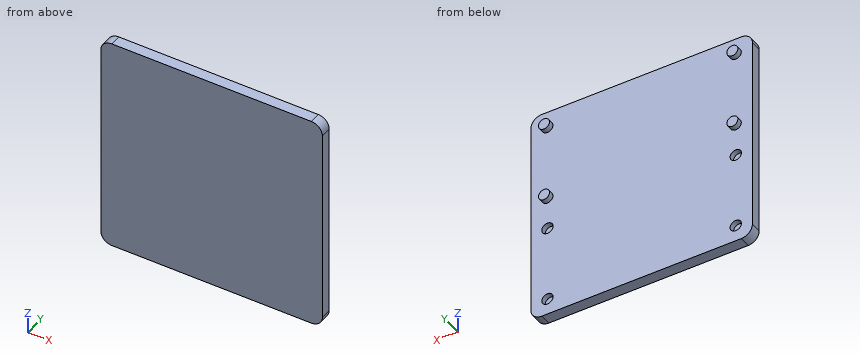
from build123d import *

# Parameters (mm, degrees)
SKETCH_1_W          = 200
SKETCH_1_H          = 200
EXTRUDE_1_DEPTH     = 10
SKETCH_2_R          = 5
EXTRUDE_2_DEPTH     = 5
FILLET_1_R          = 10
SKETCH_3_R          = 5.1
CUT_EXTRUDE_1_DEPTH = 5


with BuildPart() as part:
    # ｽｹｯﾁ1 → ﾎﾞｽ - 押し出し1 (new body)
    with BuildSketch(Plane(origin=(0, 0, 0), x_dir=(1, 0, 0), z_dir=(0, 1, 0))):
        Rectangle(SKETCH_1_W, SKETCH_1_H)
    extrude(amount=EXTRUDE_1_DEPTH)

    # ｽｹｯﾁ2 → ﾎﾞｽ - 押し出し2 (add)
    with BuildSketch(Plane(origin=(0, 10, 0), x_dir=(1, 0, 0), z_dir=(0, 1, 0))):
        with Locations(Location((-85, -15, 0), (0, 0, 90))):
            Circle(SKETCH_2_R)
        with Locations(Location((-85, -85, 0), (0, 0, 90))):
            Circle(SKETCH_2_R)
        with Locations(Location((85, -85, 0), (0, 0, 90))):
            Circle(SKETCH_2_R)
        with Locations(Location((85, -15, 0), (0, 0, 90))):
            Circle(SKETCH_2_R)
    extrude(amount=EXTRUDE_2_DEPTH)

    # ﾌｨﾚｯﾄ1
    fillet_1_edges = [part.edges().sort_by_distance(p)[0] for p in [
        (100, 5, 100),
        (-100, 5, 100),
        (-100, 5, -100),
        (100, 5, -100),
    ]]
    fillet(fillet_1_edges, radius=FILLET_1_R)

    # ｽｹｯﾁ3 → ｶｯﾄ - 押し出し1 (cut)
    with BuildSketch(Plane(origin=(0, 10, 0), x_dir=(1, 0, 0), z_dir=(0, 1, 0))):
        with Locations(Location((-85, 85, 0), (0, 0, 270))):
            Circle(SKETCH_3_R)
        with Locations(Location((85, 85, 0), (0, 0, 270))):
            Circle(SKETCH_3_R)
        with Locations(Location((-85, 15, 0), (0, 0, 270))):
            Circle(SKETCH_3_R)
        with Locations(Location((85, 15, 0), (0, 0, 270))):
            Circle(SKETCH_3_R)
    extrude(amount=-CUT_EXTRUDE_1_DEPTH, mode=Mode.SUBTRACT)


solid = part.part
The listing builds one solid part. Answer for the finished solid, in the listing's coordinates (mm). Coordinates: 2 decimals unless noted, no trailing zeros. Order: outer loops, then holes, each group sorted by start corner. A loop starts at its lowest first (then second) coordinate and runs counter-clockwise, first axis right, second up.
Q1. Consider line 1 (X direction, y = 8.6, z = -85); line 2 (Y direction, x = 46.5, z = -71); line 3 (Z direction, x = -86.5, y = 8.75). Determine where each line is inside the solid, lowest interval first.
Q2. A cutting plane is placed at A-A, the plane z = 85. Write down the section's boundary in (x, y).
Q3. A cutting plane is placed at D-D, the plane z = 53. Write down the section's boundary in (x, y).
Q4. Given P1, Ø2, axis at x = -35, z = -51.5, coming from the -Y side; P2, Ø11, axis at x = -85.5, z = -16.5, coming from the +Y side; P3, Ø5, axis at x = 85.5, z = -85.5, coming from the +Y side; P4, Ø5, axis at x = -78.5, y = 13, coming from the +Z side, each flat-ended and moving along its own axis, determine where each tip first touches the part or whether it passes through.
Q5. A cutting plane is placed at B-B, the plane x = 52. Write down the section's boundary in (y, z).
Q6. A cutting plane is placed at C-C, the plane z = -85. Write down the section's boundary in (x, y).
Answers follow:
1. line 1: x = -100 to -90.1, -79.9 to 79.9, 90.1 to 100
1. line 2: y = 0 to 10
1. line 3: z = -100 to -89.87, -80.13 to -19.87, -10.13 to 100
2. outline: (-100, 0) - (100, 0) - (100, 10) - (90, 10) - (90, 15) - (80, 15) - (80, 10) - (-80, 10) - (-80, 15) - (-90, 15) - (-90, 10) - (-100, 10) - close
3. outline: (-100, 0) - (100, 0) - (100, 10) - (-100, 10) - close
4. P1: stops at y = 0
4. P2: stops at y = 10
4. P3: stops at y = 5
4. P4: stops at z = 88
5. outline: (0, -100) - (10, -100) - (10, 100) - (0, 100) - close
6. outline: (-100, 0) - (100, 0) - (100, 10) - (90.1, 10) - (90.1, 5) - (79.9, 5) - (79.9, 10) - (-79.9, 10) - (-79.9, 5) - (-90.1, 5) - (-90.1, 10) - (-100, 10) - close
